```python
from build123d import *

# Parameters (mm, degrees)
F0_R     = 30
F0_R_2   = 82.5
F3_DEPTH = 15
F4_R     = 82.5
F4_R_2   = 30
F5_DEPTH = 15


with BuildPart() as f2:
    # F2: sweep along a path in F1
    with BuildLine(Plane.YZ) as f2_path:
        Line((0, 0), (-200, 0))
        Line((-200, 0), (-200, -390))
        Line((-200, -390), (-850, -390))
    # F0 (on Front) → F2 (sweep)
    with BuildSketch(Plane.XZ):
        Circle(F0_R)
    sweep(path=f2_path.line, transition=Transition.RIGHT)

    # F0 (on Front) → F3 (join)
    with BuildSketch(Plane.XZ):
        Circle(F0_R_2)
        Circle(F0_R, mode=Mode.SUBTRACT)
    extrude(amount=F3_DEPTH)

    # F4 (on face) → F5 (join)
    with BuildSketch(Plane.XZ.offset(850)):
        with Locations((0, -390)):
            Circle(F4_R)
        with Locations((0, -390)):
            Circle(F4_R_2, mode=Mode.SUBTRACT)
    extrude(amount=-F5_DEPTH)


solid = f2.part
```
Check sheet for the modelled part. Datum: model origin and axes. Units: mm. A direction names the side the tool comes from. Round coordinates to 2 decimals unless told otherwise and drop trailing zeros. Order: outer loops, then holes, each group sorted by start corner. A loop starts at its lowest first (then second) coordinate and runs counter-clockwise, first axis right, second up.
1) Section check C-C (y = -200). Record the boundary of the cut face in (x, z).
2) Tool access check on faces 1 (the cylindrical face through (-6.503, -507.155, -419.287)), 2 (the flat face through (-1, -850, -389)). Record the directions out of +Z, -Z, +X, -X, +Y, -Y that give a thin tool (end or side, any length) a straight path to the whole face; none if there is none.
3) Mould release check, pull along Y, two halves, no side actions. Record for faces 3 (the cylindrical face through (-3.905, -100.116, 29.745)), 4 (the cylindrical face through (-17.88, -842.6, -470.54)), 5 (the flat face through (-1, 0, 1)): +Y half, -Y half, draft (parallel to the pull), parting line (faces both ways), or undercut.
4) Scan lines: line 1 (Y direction, x = -35, z = -445.5); line 2 (Y direction, x = 49.5, z = 54.5); line 3 (Z direction, x = 5, y = -88). Record each from-to range of solid material in increasing order.
5) Go/stop test with flat-tipped pins: pin 1 Ø6 at (x, z) = (-6.5, -3.5) entering from -Y; pin 2 Ø6 at (y, z) = (-484, -396.5) entering from +X; pin 3 Ø8 at (x, z) = (-62, 5.5) entering from -Y. Record where each tip stops, or that it passes through.
6) Section check B-B (x = 0). Record the boundary of the cut face in (y, z).
7) Section check A-A (z = -390). Record the boundary of the cut face in (x, y).
8) Section check D-D (z = 0). Record the boundary of the cut face in (x, y), and give its area (3 significant figures).
Result:
1. outline: (-30, -390) arc R30 ccw to (30, -390) - (30, 0) arc R30 ccw to (-30, 0) - close
2. face 1: none
2. face 2: +Z, -Z, +X, -X, -Y
3. face 3: undercut
3. face 4: draft
3. face 5: +Y half
4. line 1: y = -850 to -835
4. line 2: y = -15 to 0
4. line 3: z = -29.58 to 29.58
5. pin 1: stops at y = -229.8
5. pin 2: stops at x = 29.8
5. pin 3: stops at y = -15
6. outline: (-850, -472.5) - (-835, -472.5) - (-835, -420) - (-170, -420) - (-170, -30) - (-15, -30) - (-15, -82.5) - (0, -82.5) - (0, 82.5) - (-15, 82.5) - (-15, 30) - (-230, 30) - (-230, -360) - (-835, -360) - (-835, -307.5) - (-850, -307.5) - close
7. outline: (-82.5, -850) - (82.5, -850) - (82.5, -835) - (30, -835) - (30, -200) arc R30 ccw to (-30, -200) - (-30, -835) - (-82.5, -835) - close
8. outline: (-82.5, -15) - (-30, -15) - (-30, -200) arc R30 ccw to (30, -200) - (30, -15) - (82.5, -15) - (82.5, 0) - (-82.5, 0) - close
8. area: 15,000 mm2
